```python
from build123d import *

# Parameters (mm, degrees)
SKETCH1_W                                      = 250
SKETCH1_H                                      = 280
BOSS_EXTRUDE1_DEPTH                            = 1.6
CSK_FOR_M5_FLAT_HEAD_MACHINE_SCREW1_AT_2_COUNT = 2
CSK_FOR_M5_FLAT_HEAD_MACHINE_SCREW1_AT_2_PITCH = 232
CSK_FOR_M5_FLAT_HEAD_MACHINE_SCREW1_AT_3_COUNT = 2
CSK_FOR_M5_FLAT_HEAD_MACHINE_SCREW1_AT_3_PITCH = 281.822639261
CSK_FOR_M5_FLAT_HEAD_MACHINE_SCREW1_AT_4_COUNT = 2
CSK_FOR_M5_FLAT_HEAD_MACHINE_SCREW1_AT_4_PITCH = 160
CSK_FOR_M3_FLAT_HEAD_MACHINE_SCREW1_AT_2_COUNT = 2
CSK_FOR_M3_FLAT_HEAD_MACHINE_SCREW1_AT_2_PITCH = 147.785317268
CSK_FOR_M3_FLAT_HEAD_MACHINE_SCREW1_AT_3_COUNT = 2
CSK_FOR_M3_FLAT_HEAD_MACHINE_SCREW1_AT_3_PITCH = 147.785317268
CSK_FOR_M3_FLAT_HEAD_MACHINE_SCREW1_AT_4_COUNT = 2
CSK_FOR_M3_FLAT_HEAD_MACHINE_SCREW1_AT_4_PITCH = 147.785317268
CSK_FOR_M3_FLAT_HEAD_MACHINE_SCREW1_AT_5_COUNT = 2
CSK_FOR_M3_FLAT_HEAD_MACHINE_SCREW1_AT_5_PITCH = 147.785317268


with BuildPart() as part:
    # Sketch1 → Boss-Extrude1 (new body)
    with BuildSketch(Plane(origin=(0, 0, 0), x_dir=(1, 0, 0), z_dir=(0, 1, 0))):
        Rectangle(SKETCH1_W, SKETCH1_H)
    extrude(amount=BOSS_EXTRUDE1_DEPTH)

    # Sketch2 → CSK for M5 Flat Head Machine Screw1 (revolve, cut)
    with BuildSketch(Plane(origin=(-116, 1.6, -80), x_dir=(0, 0, 1), z_dir=(1, 0, 0))):
        Polygon((0, 0), (0, 1.6), (2.75, 1.6), (2.75, 2.45), (5.2, 0), align=None)
    csk_for_m5_flat_head_machine_screw1 = revolve(axis=Axis((-116, 7.95, -80), (0, -1, 0)), mode=Mode.SUBTRACT)

    # CSK for M5 Flat Head Machine Screw1 at 2: CSK for M5 Flat Head Machine Screw1 ×2
    with Locations(*[(i * CSK_FOR_M5_FLAT_HEAD_MACHINE_SCREW1_AT_2_PITCH, 0, 0) for i in range(1, CSK_FOR_M5_FLAT_HEAD_MACHINE_SCREW1_AT_2_COUNT)]):
        add(csk_for_m5_flat_head_machine_screw1, mode=Mode.SUBTRACT)

    # CSK for M5 Flat Head Machine Screw1 at 3: CSK for M5 Flat Head Machine Screw1 ×2
    with Locations(*[Vector(0.8232127859153064, 0, 0.5677329558036596) * (i * CSK_FOR_M5_FLAT_HEAD_MACHINE_SCREW1_AT_3_PITCH) for i in range(1, CSK_FOR_M5_FLAT_HEAD_MACHINE_SCREW1_AT_3_COUNT)]):
        add(csk_for_m5_flat_head_machine_screw1, mode=Mode.SUBTRACT)

    # CSK for M5 Flat Head Machine Screw1 at 4: CSK for M5 Flat Head Machine Screw1 ×2
    with Locations(*[(0, 0, i * CSK_FOR_M5_FLAT_HEAD_MACHINE_SCREW1_AT_4_PITCH) for i in range(1, CSK_FOR_M5_FLAT_HEAD_MACHINE_SCREW1_AT_4_COUNT)]):
        add(csk_for_m5_flat_head_machine_screw1, mode=Mode.SUBTRACT)

    # Sketch4 → CSK for M3 Flat Head Machine Screw1 (revolve, cut)
    with BuildSketch(Plane(origin=(0, 1.6, 0), x_dir=(0, 0, 1), z_dir=(1, 0, 0))):
        Polygon((0, 0), (0, 1.6), (1.7, 1.6), (1.7, 1.45), (3.15, 0), align=None)
    csk_for_m3_flat_head_machine_screw1 = revolve(axis=Axis((0, 7.95, 0), (0, -1, 0)), mode=Mode.SUBTRACT)

    # CSK for M3 Flat Head Machine Screw1 at 2: CSK for M3 Flat Head Machine Screw1 ×2
    with Locations(*[Vector(-0.7071067811865471, 0, 0.7071067811865479) * (i * CSK_FOR_M3_FLAT_HEAD_MACHINE_SCREW1_AT_2_PITCH) for i in range(1, CSK_FOR_M3_FLAT_HEAD_MACHINE_SCREW1_AT_2_COUNT)]):
        add(csk_for_m3_flat_head_machine_screw1, mode=Mode.SUBTRACT)

    # CSK for M3 Flat Head Machine Screw1 at 3: CSK for M3 Flat Head Machine Screw1 ×2
    with Locations(*[Vector(0.7071067811865477, 0, 0.7071067811865474) * (i * CSK_FOR_M3_FLAT_HEAD_MACHINE_SCREW1_AT_3_PITCH) for i in range(1, CSK_FOR_M3_FLAT_HEAD_MACHINE_SCREW1_AT_3_COUNT)]):
        add(csk_for_m3_flat_head_machine_screw1, mode=Mode.SUBTRACT)

    # CSK for M3 Flat Head Machine Screw1 at 4: CSK for M3 Flat Head Machine Screw1 ×2
    with Locations(*[Vector(0.7071067811865477, 0, -0.7071067811865475) * (i * CSK_FOR_M3_FLAT_HEAD_MACHINE_SCREW1_AT_4_PITCH) for i in range(1, CSK_FOR_M3_FLAT_HEAD_MACHINE_SCREW1_AT_4_COUNT)]):
        add(csk_for_m3_flat_head_machine_screw1, mode=Mode.SUBTRACT)

    # CSK for M3 Flat Head Machine Screw1 at 5: CSK for M3 Flat Head Machine Screw1 ×2
    with Locations(*[Vector(-0.7071067811865478, 0, -0.7071067811865474) * (i * CSK_FOR_M3_FLAT_HEAD_MACHINE_SCREW1_AT_5_PITCH) for i in range(1, CSK_FOR_M3_FLAT_HEAD_MACHINE_SCREW1_AT_5_COUNT)]):
        add(csk_for_m3_flat_head_machine_screw1, mode=Mode.SUBTRACT)


solid = part.part
```
Input: part model. Units: mm. Frame: model coordinates. Round coordinates to 2 decimals unless told otherwise and drop trailing zeros. Loops run counter-clockwise (first coordinate to the right, second up) from the corner with the lowest first, then second, coordinate; pieces in that order, holes last. Notation, with made-up numbers: M 51,-24.75 L 73,-24.75 A14 ccw 73,-7.75 Z; hole C 82,43.5 d8. An arc over 180 degrees is marked long. Answer in a Markdown table with one row per item. Add a question column.
1. Ray query, probe 1 along Z at (x, y) = (-104.5, 0.05); probe 2 along X at (y, z) = (0.1, -104.5); probe 3 along X at (y, z) = (0.1, -77.5). Return the intervals inside material, ascending.
2. Section A-A (x = 116). Output: boundary loops of the cut face in (y, z).
3. Section B-B (z = -80). Output: boundary loops of the cut face in (x, y).
4. Contact query for a flat-ended pin moving along its axis: pin 1 (5.5 mm diameter, centred on x = -104.5, z = -104.5, fed in from +Y). Output: stop coordinate, or through.
Values follow:
| question | item | result |
|---|---|---|
| 1 | probe 1 | -140 to -106.2, -102.8 to 102.8, 106.2 to 140 |
| 1 | probe 2 | -125 to -106.2, -102.8 to 102.8, 106.2 to 125 |
| 1 | probe 3 | -125 to -118.73, -113.27 to 113.27, 118.73 to 125 |
| 2 | outline | M 0,-140 L 1.6,-140 L 1.6,-85.2 L 0,-83.6 Z; M 0,-76.4 L 1.6,-74.8 L 1.6,74.8 L 0,76.4 Z; M 0,83.6 L 1.6,85.2 L 1.6,140 L 0,140 Z |
| 3 | outline | M -125,0 L -119.6,0 L -121.2,1.6 L -125,1.6 Z; M -112.4,0 L 112.4,0 L 110.8,1.6 L -110.8,1.6 Z; M 119.6,0 L 125,0 L 125,1.6 L 121.2,1.6 Z |
| 4 | pin 1 | y = 1.2 |
